Could you check a few things on this drawing? It's one solid part, dimensions in mm from its lowest x, y, z. Give positions to 0.01 mm unless a question says otherwise; leave off trailing zeros. Order: outer loops, then holes, each group sorted by start corner. A loop starts at its lowest first (then second) coordinate and runs counter-clockwise, first axis right, second up. Notation, with made-up numbers: (74.25, 48) - (79.25, 48) arc R17 ccw to (79.25, 74) - close; hole circle Ø2 at (12, 72). An arc over 180 degrees is marked (long way). Return JSON: item names as keys, results as strings.
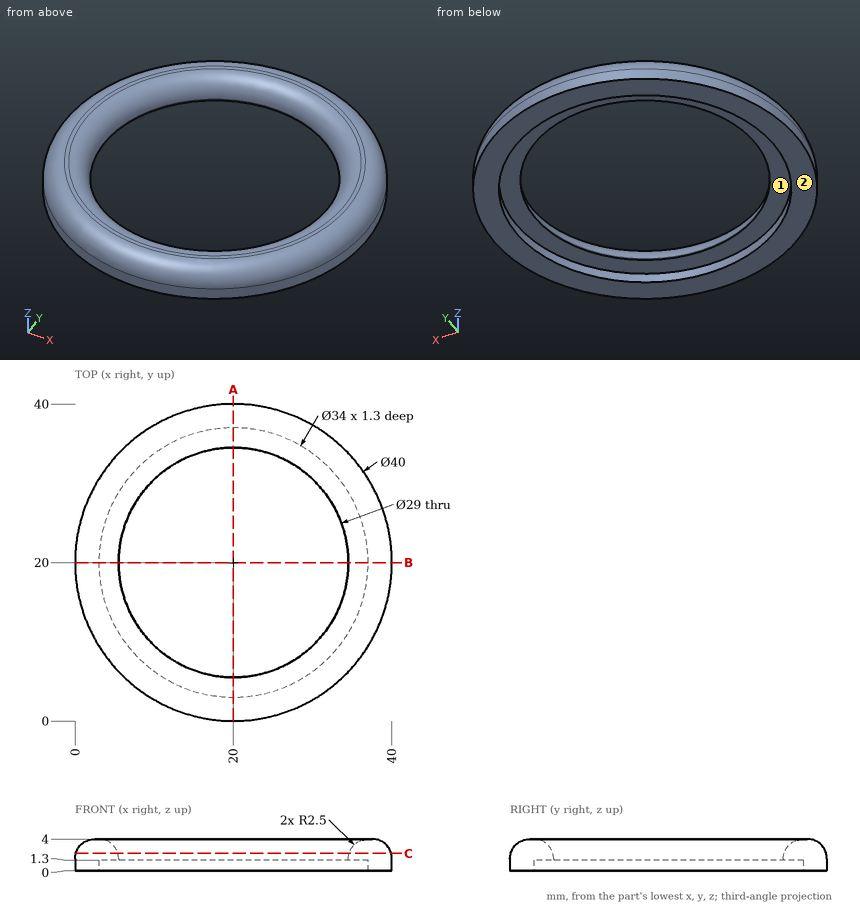
1. Suppose I cut it at C-C (z = 2.2). List the corners of the cut face in (x, y) for me, plus the area to 3 significant figures.
Checks:
{"outline": "circle Ø39.8 at (20, 20); hole circle Ø29.2 at (20, 20)", "area": "574 mm^2"}
2. Thinking about a two-plate mould opening in Y: for the marked faces 1 and 2, which applies, +Y half, -Y half, draft (parallel to the pull), parting line (faces both ways), or undercut?
Checks:
{"face 1": "undercut", "face 2": "draft"}
3. If I drill on L1, parallel to Y at x = 20, z = 1.4; L2, parallel to Y at x = 20, z = 0.75; L3, parallel to X at y = 17, z = 3.25, over which ranges is the centre line in solid material (lowest first)? Write a range as [from, to].
Checks:
{"L1": "[0, 5.5], [34.5, 40]", "L2": "[0, 3], [37, 40]", "L3": "[0.95, 5.08], [34.92, 39.05]"}
4. Suppose I cut it at A-A (x = 20). List the corners of the cut face in (y, z) for me.
Checks:
{"outline": "(0, 0) - (3, 0) - (3, 1.3) - (5.5, 1.3) - (5.5, 1.5) arc R2.5 ccw to (3, 4) - (2.5, 4) arc R2.5 ccw to (0, 1.5) - close; (34.5, 1.3) - (37, 1.3) - (37, 0) - (40, 0) - (40, 1.5) arc R2.5 ccw to (37.5, 4) - (37, 4) arc R2.5 ccw to (34.5, 1.5) - close"}
5. For pin 1 Ø10 at (x, y) = (13.5, 14) entering from -Z; pin 2 Ø2 at (x, y) = (33.5, 14.5) entering from -Z; pin 3 Ø1.5 at (x, z) = (32.5, 1) entering from +Y, each with a flat end and sliding along its axis, tell me the tip position at first contact or that it passes through.
Checks:
{"pin 1": "through", "pin 2": "z = 1.3", "pin 3": "y = 36.18"}
